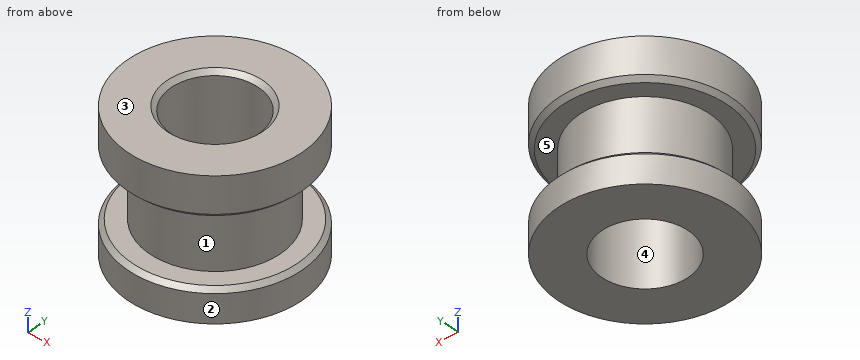
```python
from build123d import *

# Parameters (mm, degrees)
F2_SIZE = 0.4


with BuildPart() as f1:
    # F0 (on Front) → F1 (revolve)
    with BuildSketch(Plane.XZ):
        Polygon((8, 3), (8, 6.7), (4, 6.7), (4, -6), (8, -6), (8, -3), (6, -3), (6, 3), align=None)
    revolve(axis=Axis((0, 0, 0), (0, 0, 1)))

    # F2
    f2_edges = [f1.edges().sort_by_distance(p)[0] for p in [
        (-8, 0, 3),
        (-8, 0, -3),
        (-4, 0, 6.7),
    ]]
    chamfer(f2_edges, length=F2_SIZE)


solid = f1.part
```
The listing builds one solid part. Answer for the finished solid, in the listing's coordinates (mm). Face numbers are marked on the shaded views. A direction names the side the tool comes from. Coordinates: 2 decimals unless noted, no trailing zeros. Write each loop counter-clockwise with the first axis right and the second up, starting at its lowest first coordinate (ties: lowest second). Pieces come first, ordered by that corner, then holes.
Q1. The mould has two halves that part along Z. Classify the marked faces 3, 4 and 5: released by +Z, released by -Z, zero draft, split by the parting line, or undercut.
Returned:
face 3: released by +Z
face 4: zero draft
face 5: undercut
Q2. Which of the six approach directions +Z, -Z, +X, -X, +Y, -Y give full straight-line access (tool end or side, diameter ignored) to the marked faces 1 and 2?
Returned:
face 1: none
face 2: +Z, -Z
Q3. Given P1, Ø1.5, axis at x = 1.5, z = 4, coming from the -Y side; P2, Ø4, axis at x = 0.5, y = 0, coming from the +Z side; P3, Ø4.5, axis at x = -2, y = 0.5, coming from the +Z side; P4, Ø5, axis at x = -2, z = -1, coming from the +Y side, each flat-ended and moving along its own axis, determine where each tip first touches the part or whether it passes through.
Returned:
P1: stops at y = -7.96
P2: passes through
P3: stops at z = 6.61
P4: stops at y = 7.89
Q4. Section C-C, the plane z = 4.75 is taken. Write down the section's boundary in (x, y), then the cut area to 3 significant figures.
Returned:
outline: circle Ø16 at (0, 0); hole circle Ø8 at (0, 0)
area: 151 mm2
Q5. Section A-A, the plane x = 0 is taken. Write down the section's boundary in (y, z).
Returned:
outline: (-8, -6) - (-4, -6) - (-4, 6.3) - (-4.4, 6.7) - (-8, 6.7) - (-8, 3.4) - (-7.6, 3) - (-6, 3) - (-6, -3) - (-7.6, -3) - (-8, -3.4) - close; (4, -6) - (8, -6) - (8, -3.4) - (7.6, -3) - (6, -3) - (6, 3) - (7.6, 3) - (8, 3.4) - (8, 6.7) - (4.4, 6.7) - (4, 6.3) - close
Q6. Find the intervals of material crossed by line 1 along Z through (x, y) = (0.25, 7.5); line 2 along Y through (x, z) = (0, 2.25); line 3 along Y through (x, z) = (0, -3.5), in increasing order.
Returned:
line 1: z = -6 to -3, 3 to 6.7
line 2: y = -6 to -4, 4 to 6
line 3: y = -8 to -4, 4 to 8
